from build123d import *

# Parameters (mm, degrees)
SKETCH1_R           = 8.18
BOSS_EXTRUDE1_DEPTH = 8
CUT_EXTRUDE1_DEPTH  = 9
CIRPATTERN1_COUNT   = 11
SKETCH4_R           = 9.68
BOSS_EXTRUDE2_DEPTH = 1
SKETCH6_R           = 2
CUT_EXTRUDE2_DEPTH  = 11


with BuildPart() as part:
    # Sketch1 → Boss-Extrude1 (new body)
    with BuildSketch(Plane(origin=(0, 0, 0), x_dir=(0, 0, -1), z_dir=(1, 0, 0))):
        Circle(SKETCH1_R)
    extrude(amount=BOSS_EXTRUDE1_DEPTH)

    # Sketch2 → Cut-Extrude1 (cut, through all)
    with BuildSketch(Plane(origin=(0, 0, 0), x_dir=(0, 0, -1), z_dir=(1, 0, 0))):
        with BuildLine():
            ThreePointArc((0, 6.1), (0.961072859, 6.586806473), (1.347953386, 7.592274046))
            ThreePointArc((1.347953386, 7.592274046), (1.511589464, 7.896914613), (1.85, 7.96805497))
            ThreePointArc((1.85, 7.96805497), (0, 8.18), (-1.85, 7.96805497))
            ThreePointArc((-1.85, 7.96805497), (-1.511589464, 7.896914613), (-1.347953386, 7.592274046))
            ThreePointArc((-1.347953386, 7.592274046), (-0.961072859, 6.586806473), (0, 6.1))
        make_face()
    cut_extrude1 = extrude(amount=CUT_EXTRUDE1_DEPTH, mode=Mode.SUBTRACT)

    # CirPattern1: Cut-Extrude1 ×11 about axis
    cirpattern1_axis = Axis((0, 0, 0), (1, 0, 0))
    for i in range(1, CIRPATTERN1_COUNT):
        add(cut_extrude1.rotate(cirpattern1_axis, i * 360 / CIRPATTERN1_COUNT), mode=Mode.SUBTRACT)

    # Sketch4 → Boss-Extrude2 (add)
    with BuildSketch(Plane.ZY):
        Circle(SKETCH4_R)
    boss_extrude2 = extrude(amount=BOSS_EXTRUDE2_DEPTH)

    # Mirror1: Boss-Extrude2 across plane
    add(boss_extrude2.mirror(Plane.ZY.offset(-4)))

    # Sketch6 → Cut-Extrude2 (cut, through all)
    with BuildSketch(Plane.ZY.offset(1)):
        Circle(SKETCH6_R)
    extrude(amount=-CUT_EXTRUDE2_DEPTH, mode=Mode.SUBTRACT)


solid = part.part
Check sheet for the modelled part. Datum: model origin and axes. Units: mm. A direction names the side the tool comes from. Round coordinates to 2 decimals unless told otherwise and drop trailing zeros. Order: outer loops, then holes, each group sorted by start corner. A loop starts at its lowest first (then second) coordinate and runs counter-clockwise, first axis right, second up.
(1) Cross-section at C-C, the plane y = 3.25. Enter the section's corners in (x, z).
(2) Cross-section at A-A, the plane y = 0. Enter the section's corners in (x, z).
(3) Access from +Z, -Z, +X, -X, +Y, -Y to the whole of each face (thin tool, end or side, straight path). Record for faces 1 (the cylindrical face through (3.944, 5.018, -4.355)), 2 (the cylindrical face through (3.94, -6.04, 2.76)), 3 (the cylindrical face through (3.944, 0.022, -6.669)), 4 (the cylindrical face through (3.944, 3.625, -5.599)), 5 (the cylindrical face through (3.94, 7.85, 2.3)).
(4) Cross-section at B-B, the plane x = 8.5. Enter the section's corners in (y, z).
(5) Draft check along Z on faces 6 (the cylindrical face through (3.944, -3.392, 7.444)), 7 (the cylindrical face through (3.944, 1.857, 6.406)), 8 (the cylindrical face through (3.94, -6.6, 0.93)), 9 (the flat face through (9, 2.3, -0.1)). Enter one of: pulls with the +Z half, pulls with the -Z half, needs draft (parallel to the pull), parting line crosses it, or undercut.
(6) Cross-section at D-D, the plane y = 8.75. Enter the section's corners in (x, z).
(7) Scan lines: probe 1 along X at (y, z) = (-4, -8); probe 2 along Z at (x, y) = (7.5, -6.5); probe 3 along Z at (x, y) = (6.25, -7). Record each from-to range of solid material in increasing order.
(8) Go/stop test with flat-tipped pins: P1, Ø4, axis at x = 3.5, z = -2, coming from the +Y side; P2, Ø3, axis at x = 2, y = -7.5, coming from the -Z side; P3, Ø3, axis at x = 0.5, y = 5, coming from the -Z side. Record where each tip stops, or that it passes through.
Check sheet entries:
1. outline: (-1, -9.12) - (0, -9.12) - (0, -5.49) - (8, -5.49) - (8, -9.12) - (9, -9.12) - (9, 9.12) - (8, 9.12) - (8, 5.49) - (0, 5.49) - (0, 9.12) - (-1, 9.12) - close
2. outline: (-1, -9.68) - (0, -9.68) - (0, -6.64) - (8, -6.64) - (8, -9.68) - (9, -9.68) - (9, -2) - (-1, -2) - close; (-1, 2) - (9, 2) - (9, 9.68) - (8, 9.68) - (8, 6.64) - (0, 6.64) - (0, 9.68) - (-1, 9.68) - close
3. face 1: +Y
3. face 2: -Y
3. face 3: none
3. face 4: -Z
3. face 5: +Z, +Y
4. outline: circle Ø19.36 at (0, 0); hole circle Ø4 at (0, 0)
5. face 6: pulls with the +Z half
5. face 7: undercut
5. face 8: undercut
5. face 9: needs draft
6. outline: (-1, -4.14) - (0, -4.14) - (0, 4.14) - (-1, 4.14) - close; (8, -4.14) - (9, -4.14) - (9, 4.14) - (8, 4.14) - close
7. probe 1: x = -1 to 0, 8 to 9
7. probe 2: z = -4.92 to -3.24, -0.98 to 0.98, 3.24 to 4.92
7. probe 3: z = -4.23 to -3.48, -0.8 to 0.8, 3.48 to 4.23
8. P1: stops at y = 7.98
8. P2: stops at z = -4.98
8. P3: stops at z = -8.99
